Work out the finished part from the listing and answer in its coordinate system (mm). Face numbers are marked on the shaded views. A direction names the side the tool comes from. Round coordinates to 2 decimals unless told otherwise and drop trailing zeros. Order: outer loops, then holes, each group sorted by start corner. A loop starts at its lowest first (then second) coordinate and runs counter-clockwise, first axis right, second up. Notation, with made-up numbers: (83.5, -27) - (124.5, -27) arc R15 ccw to (124.5, -15) - close; hole circle Ø7 at (9, 55). An arc over 180 degrees is marked (long way). Answer in a Markdown table with one row per item.
from build123d import *

# Parameters (mm, degrees)
BOSS_EXTRUDE1_DEPTH     = 70
CUT_EXTRUDE3_DEPTH      = 145.019444896
CUT_EXTRUDE3_DEPTH_BACK = 145.019444896
SKETCH2_W               = 40
SKETCH2_H               = 90
CUT_EXTRUDE4_DEPTH      = 145.019444896
CUT_EXTRUDE4_DEPTH_BACK = 145.019444896
SKETCH3_W               = 74.200339426
SKETCH3_H               = 40


with BuildPart() as part:
    # Sketch1 → Boss-Extrude1 (new body)
    with BuildSketch(Plane.XY):
        with BuildLine():
            Line((0, 3), (-67.156880159, 3))
            ThreePointArc((-67.156880159, 3), (-70.33029352, 4.564954284), (-71.020583464, 8.03527618))
            Line((-71.020583464, 8.03527618), (-51.873686922, 79.492466883))
            ThreePointArc((-51.873686922, 79.492466883), (-48.532088385, 82.422970148), (-44.545882001, 80.457190703))
            Line((-44.545882001, 80.457190703), (-18.49562947, 35.336829768))
            ThreePointArc((-18.49562947, 35.336829768), (-16.066804035, 33.473126463), (-13.031527854, 33.872728153))
            Line((-13.031527854, 33.872728153), (-1.828193725, 40.340976128))
            ThreePointArc((-1.828193725, 40.340976128), (-0.36409211, 41.805077743), (0.171806275, 43.805077743))
            Line((0.171806275, 43.805077743), (0.171806275, 64.29182561))
            ThreePointArc((0.171806275, 64.29182561), (-2.828193725, 66.625142685), (-5.828193725, 64.29182561))
            Line((-5.828193725, 64.29182561), (-5.828193725, 47.269179358))
            ThreePointArc((-5.828193725, 47.269179358), (-6.36409211, 45.269179358), (-7.828193725, 43.805077743))
            Line((-7.828193725, 43.805077743), (-10.835375432, 42.068880575))
            ThreePointArc((-10.835375432, 42.068880575), (-13.870651612, 41.669278885), (-16.299477047, 43.53298219))
            Line((-16.299477047, 43.53298219), (-46.592370266, 96.001812354))
            ThreePointArc((-46.592370266, 96.001812354), (-50.57857665, 97.967591799), (-53.920175186, 95.037088534))
            Line((-53.920175186, 95.037088534), (-78.839935701, 2.03527618))
            ThreePointArc((-78.839935701, 2.03527618), (-78.149645757, -1.435045716), (-74.976232396, -3))
            Line((-74.976232396, -3), (0, -3))
            ThreePointArc((0, -3), (3, 0), (0, 3))
        make_face()
    extrude(amount=BOSS_EXTRUDE1_DEPTH)

    # Sketch2 → Cut-Extrude3 (cut, two sides: drawn at the far end of the back side and taken through both)
    with BuildSketch(Plane(origin=(0, 0, 0), x_dir=(0, 0, -1), z_dir=(1, 0, 0)).offset(-CUT_EXTRUDE3_DEPTH_BACK)):
        with Locations((-35.588760561, 57.237154529)):
            Rectangle(SKETCH2_W, SKETCH2_H)
    extrude(amount=CUT_EXTRUDE3_DEPTH + CUT_EXTRUDE3_DEPTH_BACK, mode=Mode.SUBTRACT)

    # Sketch3 → Cut-Extrude4 (cut, two sides: drawn at the far end of the back side and taken through both)
    with BuildSketch(Plane(origin=(0, 0, 0), x_dir=(1, 0, 0), z_dir=(0, 1, 0)).offset(-CUT_EXTRUDE4_DEPTH_BACK)):
        with Locations((-46.354271726, -36.051698815)):
            Rectangle(SKETCH3_W, SKETCH3_H)
    extrude(amount=CUT_EXTRUDE4_DEPTH + CUT_EXTRUDE4_DEPTH_BACK, mode=Mode.SUBTRACT)


solid = part.part
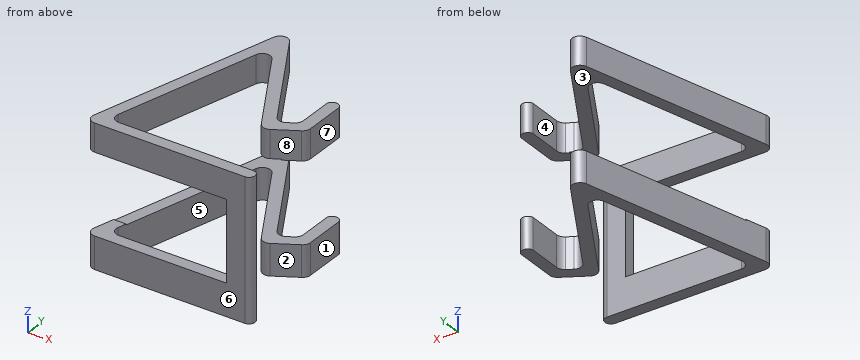
1) Find the intervals of material crossed by probe 1 along X at (y, z) = (59, 57.5); probe 2 along X at (y, z) = (71, 14); probe 3 along Y at (x, z) = (-8.5, 57), in increasing order. Write a range as from..to.
Filled in:
| item | result |
|---|---|
| probe 1 | x = -63.58..-57.36, -32.16..-25.23, -5.83..0.17 |
| probe 2 | x = -60.36..-54.15, -39.09..-32.16 |
| probe 3 | y = -3..3, 36.49..43.42 |
2) The mould has two halves that part along Y. Classify the marked faces 6, 7 and 8: released by +Y, released by -Y, zero draft, split by the parting line, or undercut.
Filled in:
| item | result |
|---|---|
| face 6 | released by -Y |
| face 7 | zero draft |
| face 8 | undercut |
3) Which of the six approach directions +Z, -Z, +X, -X, +Y, -Y give full straight-line access (tool end or side, diameter ignored) to the marked faces 1, 2, 3, 4 and 5?
Filled in:
| item | result |
|---|---|
| face 1 | +Z, -Z, +X, +Y |
| face 2 | +Z, -Z, +X |
| face 3 | -X, +Y, -Y |
| face 4 | +Z, -Z, +Y |
| face 5 | +Z, -Z |
4) Each of these flat-tipped pins is pushed along its axis until it touches: pin 1 (4 mm diameter, centred on x = -56, y = 54.5, fed in from +Z); pin 2 (12 mm diameter, centred on x = -61.5, y = 63.5, fed in from -Z); pin 3 (11.5 mm diameter, centred on y = 57.5, z = 62.5, fed in from +X); pin 4 (11.5 mm diameter, centred on y = 58, z = 65.5, fed in from -X). Where does it stop, or does it pass through?
Filled in:
| item | result |
|---|---|
| pin 1 | passes through |
| pin 2 | stops at z = 0 |
| pin 3 | stops at x = 0.17 |
| pin 4 | stops at x = -65.38 |
5) Find section C-C, the plane y = 19.5. Give the vertices of the cut face in (x, z).
Filled in:
| item | result |
|---|---|
| outline | (-74.16, 0) - (-67.95, 0) - (-67.95, 15.59) - (-74.16, 15.59) - close; (-74.16, 56.05) - (-67.95, 56.05) - (-67.95, 70) - (-74.16, 70) - close |
6) Find section B-B, the plane y = 69.5. Give the vertices of the cut face in (x, z).
Filled in:
| item | result |
|---|---|
| outline | (-60.76, 0) - (-54.55, 0) - (-54.55, 15.59) - (-60.76, 15.59) - close; (-60.76, 56.05) - (-54.55, 56.05) - (-54.55, 70) - (-60.76, 70) - close; (-38.22, 0) - (-31.29, 0) - (-31.29, 15.59) - (-38.22, 15.59) - close; (-38.22, 56.05) - (-31.29, 56.05) - (-31.29, 70) - (-38.22, 70) - close |
7) Find section A-A, the plane z = 12.5. Give the vertices of the cut face in (x, y), then the cut area to 3 significant figures.
Filled in:
| item | result |
|---|---|
| outline | (-78.84, 2.04) arc R4 ccw to (-74.98, -3) - (0, -3) arc R3 ccw to (0, 3) - (-67.16, 3) arc R4 cw to (-71.02, 8.04) - (-51.87, 79.49) arc R4 cw to (-44.55, 80.46) - (-18.5, 35.34) arc R4 ccw to (-13.03, 33.87) - (-1.83, 40.34) arc R4 ccw to (0.17, 43.81) - (0.17, 64.29) arc R3.1 ccw to (-5.83, 64.29) - (-5.83, 47.27) arc R4 cw to (-7.83, 43.81) - (-10.84, 42.07) arc R4 cw to (-16.3, 43.53) - (-46.59, 96) arc R4 ccw to (-53.92, 95.04) - close |
| area | 1,720 mm^2 |
8) Find section D-D, the plane y = 0. Give the vertices of the cut face in (x, z), then the cut area to 3 significant figures.
Filled in:
| item | result |
|---|---|
| outline | (-78.85, 0) - (3, 0) - (3, 70) - (-78.85, 70) - (-78.85, 56.05) - (-9.25, 56.05) - (-9.25, 16.05) - (-78.85, 16.05) - close |
| area | 2,950 mm^2 |
